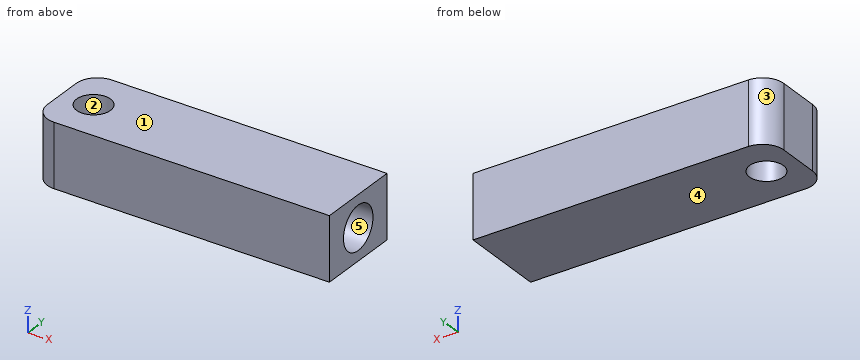
```python
from build123d import *

# Parameters (mm, degrees)
SKETCH_2_R          = 1.6
EXTRUDE_1_DEPTH     = 6
SKETCH_3_R          = 2.05
CUT_EXTRUDE_1_DEPTH = 20


with BuildPart() as part:
    # 草图2 → 凸台-拉伸1 (new body)
    with BuildSketch(Plane.XY):
        with BuildLine():
            Line((0, 2), (0, 6))
            ThreePointArc((0, 6), (0.585786438, 7.414213562), (2, 8))
            Line((2, 8), (28, 8))
            Line((28, 8), (28, 0))
            Line((28, 0), (2, 0))
            ThreePointArc((2, 0), (0.585786438, 0.585786438), (0, 2))
        make_face()
        with Locations((3, 4)):
            Circle(SKETCH_2_R, mode=Mode.SUBTRACT)
    extrude(amount=EXTRUDE_1_DEPTH)

    # 草图3 → 切除-拉伸1 (cut)
    with BuildSketch(Plane(origin=(28, 0, 0), x_dir=(0, 0, -1), z_dir=(1, 0, 0))):
        with Locations((-3, 4)):
            Circle(SKETCH_3_R)
    extrude(amount=-CUT_EXTRUDE_1_DEPTH, mode=Mode.SUBTRACT)


solid = part.part
```
Geometry check sheet. Reference: the model listing, model coordinates, mm. Face numbers are marked on the shaded views. A direction names the side the tool comes from. Coordinates: 2 decimals unless noted, no trailing zeros. Loops run counter-clockwise (first coordinate to the right, second up) from the corner with the lowest first, then second, coordinate; pieces in that order, holes last.
Item 1: Sectioned sample at B-B, the plane y = 4. Record the boundary of the cut face in (x, z).
Item 2: Thickness scan on line 1 (Y direction, x = 3, z = 4.7); line 2 (Y direction, x = 19, z = 3); line 3 (Z direction, x = 10.25, y = 4.75). Record the ranges inside material, lowest first.
Item 3: Release check for a two-part mould opening along Y. For the marked faces 1, 2 and 3 record: released by +Y, released by -Y, zero draft, split by the parting line, or undercut.
Item 4: Go/stop test with a flat-tipped pin: pin 1 Ø2 at (y, z) = (3.5, 2.5) entering from +X. Record where the tip stops, or that it passes through.
Item 5: Sectioned sample at A-A, the plane x = 3. Record the boundary of the cut face in (y, z).
Item 6: Access from +Z, -Z, +X, -X, +Y, -Y to the whole of each face (thin tool, end or side, straight path). Record for the marked faces 4 and 5.
Item 7: Sectioned sample at C-C, the plane z = 3. Record the boundary of the cut face in (x, y), then the cut area to 3 significant figures.
Item 8: Sectioned sample at D-D, the plane x = 24.25. Record the boundary of the cut face in (y, z), then the cut area to 3 significant figures.
Check result:
1. outline: (0, 0) - (1.4, 0) - (1.4, 6) - (0, 6) - close; (4.6, 0) - (28, 0) - (28, 0.95) - (8, 0.95) - (8, 5.05) - (28, 5.05) - (28, 6) - (4.6, 6) - close
2. line 1: y = 0 to 2.4, 5.6 to 8
2. line 2: y = 0 to 1.95, 6.05 to 8
2. line 3: z = 0 to 1.09, 4.91 to 6
3. face 1: zero draft
3. face 2: undercut
3. face 3: released by +Y
4. pin 1: stops at x = 8
5. outline: (0, 0) - (2.4, 0) - (2.4, 6) - (0, 6) - close; (5.6, 0) - (8, 0) - (8, 6) - (5.6, 6) - close
6. face 4: -Z, +X, -X, +Y, -Y
6. face 5: +X
7. outline: (0, 2) arc R2 ccw to (2, 0) - (28, 0) - (28, 1.95) - (8, 1.95) - (8, 6.05) - (28, 6.05) - (28, 8) - (2, 8) arc R2 ccw to (0, 6) - close; hole circle Ø3.2 at (3, 4)
7. area: 132 mm2
8. outline: (0, 0) - (8, 0) - (8, 6) - (0, 6) - close; hole circle Ø4.1 at (4, 3)
8. area: 34.8 mm2
